Autodesk Inventor part; units mm, degrees
ref_plane "YZ Plane" through (0, 0, 0) normal (1, 0, 0) x (0, 1, 0)
ref_plane "XZ Plane" through (0, 0, 0) normal (0, 1, 0) x (-1, 0, 0)
ref_plane "XY Plane" through (0, 0, 0) normal (0, 0, 1) x (1, 0, 0)
sketch "BaseI" plane through (0, 0, 0) normal (0, 0, 1) x (1, 0, 0)
  line L0 (-4.5, -10) -> (-2.65, -10)
  line L1 (5, -9.5) -> (5, 9.5)
  line L2 (4.5, 10) -> (2.65, 10)
  line L3 (-5, 9.5) -> (-5, -9.5)
  line L4 (-5, -10) -> (5, 10) construction
  line L5 (5, -10) -> (-5, 10) construction
  line L6 (3.85, 8.5) -> (2.65, 8.5)
  line L7 (-4.15, 8.2) -> (-4.15, 5.1)
  line L8 (-3.85, 4.8) -> (-2.65, 4.8)
  line L9 (4.15, 5.1) -> (4.15, 8.2)
  line L10 (4.15, 8.5) -> (-4.15, 4.8) construction
  line L11 (-4.15, 8.5) -> (4.15, 4.8) construction
  line L12 (-1.55, 3) -> (1.55, 3)
  line L13 (2.15, 3.6) -> (2.15, 4.3)
  line L14 (-2.15, 9.5) -> (-2.15, 9)
  line L15 (-2.15, 3) -> (2.15, 10) construction
  line L16 (2.15, 3) -> (-2.15, 10) construction
  line L17 (3.85, -8.5) -> (2.65, -8.5)
  line L18 (-4.15, -8.2) -> (-4.15, -5.1)
  line L19 (-3.85, -4.8) -> (-2.65, -4.8)
  line L20 (4.15, -5.1) -> (4.15, -8.2)
  line L21 (4.15, -8.5) -> (-4.15, -4.8) construction
  line L22 (-4.15, -8.5) -> (4.15, -4.8) construction
  line L23 (1.55, -3) -> (-1.55, -3)
  line L24 (-2.15, -3.6) -> (-2.15, -4.3)
  line L25 (2.15, -9.5) -> (2.15, -9)
  line L26 (2.15, -3) -> (-2.15, -10) construction
  line L27 (-2.15, -3) -> (2.15, -10) construction
  arc A0 (-4.5, 10) -> (-5, 9.5) centre (-4.5, 9.5) ccw
  arc A1 (5, 9.5) -> (4.5, 10) centre (4.5, 9.5) ccw
  arc A2 (4.5, -10) -> (5, -9.5) centre (4.5, -9.5) ccw
  arc A3 (-5, -9.5) -> (-4.5, -10) centre (-4.5, -9.5) ccw
  line L28 (-2.65, 10) -> (-4.5, 10)
  line L29 (2.65, -10) -> (4.5, -10)
  arc A4 (-3.85, 8.5) -> (-4.15, 8.2) centre (-3.85, 8.2) ccw
  arc A5 (-4.15, 5.1) -> (-3.85, 4.8) centre (-3.85, 5.1) ccw
  arc A6 (4.15, 8.2) -> (3.85, 8.5) centre (3.85, 8.2) ccw
  arc A7 (3.85, 4.8) -> (4.15, 5.1) centre (3.85, 5.1) ccw
  arc A8 (-3.85, -4.8) -> (-4.15, -5.1) centre (-3.85, -5.1) ccw
  arc A9 (-4.15, -8.2) -> (-3.85, -8.5) centre (-3.85, -8.2) ccw
  arc A10 (4.15, -5.1) -> (3.85, -4.8) centre (3.85, -5.1) ccw
  arc A11 (3.85, -8.5) -> (4.15, -8.2) centre (3.85, -8.2) ccw
  arc A12 (-2.15, 3.6) -> (-1.55, 3) centre (-1.55, 3.6) ccw
  arc A13 (1.55, 3) -> (2.15, 3.6) centre (1.55, 3.6) ccw
  arc A14 (-1.55, -3) -> (-2.15, -3.6) centre (-1.55, -3.6) ccw
  arc A15 (2.15, -3.6) -> (1.55, -3) centre (1.55, -3.6) ccw
  arc A16 (-2.15, 9.5) -> (-2.65, 10) centre (-2.65, 9.5) ccw
  arc A17 (2.65, 10) -> (2.15, 9.5) centre (2.65, 9.5) ccw
  line L30 (-2.65, 8.5) -> (-3.85, 8.5)
  line L31 (2.65, 4.8) -> (3.85, 4.8)
  line L32 (2.15, 9) -> (2.15, 9.5)
  line L33 (-2.15, 4.3) -> (-2.15, 3.6)
  line L34 (2.15, -4.3) -> (2.15, -3.6)
  line L35 (-2.15, -9) -> (-2.15, -9.5)
  line L36 (2.65, -4.8) -> (3.85, -4.8)
  line L37 (-2.65, -8.5) -> (-3.85, -8.5)
  arc A18 (-2.15, 4.3) -> (-2.65, 4.8) centre (-2.65, 4.3) ccw
  arc A19 (2.65, 4.8) -> (2.15, 4.3) centre (2.65, 4.3) ccw
  arc A20 (2.15, 9) -> (2.65, 8.5) centre (2.65, 9) ccw
  arc A21 (-2.65, 8.5) -> (-2.15, 9) centre (-2.65, 9) ccw
  arc A22 (-2.65, -4.8) -> (-2.15, -4.3) centre (-2.65, -4.3) ccw
  arc A23 (2.15, -4.3) -> (2.65, -4.8) centre (2.65, -4.3) ccw
  arc A24 (2.65, -8.5) -> (2.15, -9) centre (2.65, -9) ccw
  arc A25 (-2.15, -9) -> (-2.65, -8.5) centre (-2.65, -9) ccw
  arc A26 (-2.65, -10) -> (-2.15, -9.5) centre (-2.65, -9.5) ccw
  arc A27 (2.15, -9.5) -> (2.65, -10) centre (2.65, -9.5) ccw
  circle A28 centre (0, 0) radius 1.65
  point P0 (0, 6.65)
  point P1 (0, 6.5)
  point P2 (0, -6.65)
  point P3 (0, -6.5)
  point P4 (0, 6.5)
  point P5 (0, 10)
  point P6 (0, -6.5)
  point P7 (0, -10)
  point P8 (0, 6.65)
  point P9 (0, 10)
  point P10 (0, 6.65)
  point P11 (0, -6.65)
  point P12 (0, -10)
  point P13 (0, -6.5)
  point P14 (0, -6.65)
  point P15 (0, 6.5)
  dimension "d0" = 10
  dimension "d1" = 20
  dimension "d2" = 7
  dimension "d3" = 4.3
  dimension "d4" = 7
  dimension "d5" = 4.3
  dimension "d6" = 8.3
  dimension "d7" = 8.3
  dimension "d8" = 3.7
  dimension "d9" = 3.7
  dimension "d10" = 1.5
  dimension "d11" = 1.5
  dimension "d12" = 0.5
  dimension "d13" = 0.3
  dimension "d14" = 0.6
  dimension "d15" = 0.5
  dimension "d16" = 0.5
  dimension "d17" = 3.3
extrude "押し出し1" add sketch "BaseI" along normal blind 40
properties part number "I330" material "アルミニウム 6061"
Geometry: final body of the model. Coordinates: model frame, mm. A direction names the side the tool comes from. Give positions to 0.01 mm unless a question says otherwise; leave off trailing zeros. Loops run counter-clockwise (first coordinate to the right, second up) from the corner with the lowest first, then second, coordinate; pieces in that order, holes last. Notation, with made-up numbers: M -36,84 L 7,84 A36 cw 7,121 Z; hole C 80.5,27 d7. An arc over 180 degrees is marked long. Put each result on its own line as item: value.
1) Reachability of faces 4 (the flat face through (5, 0, 20)), 5 (the flat face through (4.15, -7, 20)), 6 (the flat face through (0, -3, 20)) from +Z, -Z, +X, -X, +Y, -Y: full face, straight path, thin tool, end or side. Return the list, or none.
Computed values:
face 4: +Z, -Z, +X, +Y, -Y
face 5: +Z, -Z
face 6: +Z, -Z, -Y
2) Material intervals for L1, parallel to Y at x = -3, z = 17; L2, parallel to Y at x = 0, z = 27; L3, parallel to X at y = -5.75, z = 19, sorted ascending. Write a range as from..to.
Computed values:
L1: y = -10..-8.5, -4.8..4.8, 8.5..10
L2: y = -3..-1.65, 1.65..3
L3: x = -5..-4.15, 4.15..5
3) Cut plane A-A, the plane y = 0. Return the cut outline in (x, z), plus the area to 3 significant figures.
Computed values:
outline: M -5,0 L -1.65,0 L -1.65,40 L -5,40 Z; M 1.65,0 L 5,0 L 5,40 L 1.65,40 Z
area: 268 mm^2
4) Mould query, pull axis Y, two halves, no side actions, for faces 1 (the flat face through (0, 3, 20)), 2 (the flat face through (0, 2, 0)), 3 (the flat face through (-3, 8.5, 20)). Classes: released by +Y, released by -Y, zero draft, split by the parting line, or undercut.
Computed values:
face 1: released by +Y
face 2: zero draft
face 3: undercut
5) First-contact query: P1, Ø2, axis at x = -2, z = 7, coming from the -Y side. Flat tip, straight axial feed; report the tip coordinate or a pass-through.
Computed values:
P1: stops at y = -10
6) Cut plane B-B, the plane x = 0. Return the cut outline in (y, z).
Computed values:
outline: M -3,0 L -1.65,0 L -1.65,40 L -3,40 Z; M 1.65,0 L 3,0 L 3,40 L 1.65,40 Z
